Autodesk Inventor part; units mm, degrees
ref_plane "YZ Plane" through (0, 0, 0) normal (1, 0, 0) x (0, 1, 0)
ref_plane "XZ Plane" through (0, 0, 0) normal (0, 1, 0) x (-1, 0, 0)
ref_plane "XY Plane" through (0, 0, 0) normal (0, 0, 1) x (1, 0, 0)
sketch "スケッチ1" plane through (0, 0, 0) normal (1, 0, 0) x (0, 1, 0)
  circle A0 centre (0, 0) radius 10
  circle A1 centre (0, -10) radius 1.35
  circle A2 centre (8.6603, 5) radius 1.35
  circle A3 centre (-8.6603, 5) radius 1.35
  circle A4 centre (0, 0) radius 5
  line L0 (0, 0) -> (0, 50)
  circle A5 centre (0, 50) radius 22.5
  circle A6 centre (0, 0) radius 14
  line L1 (-14, 0) -> (-22.5, 50)
  line L2 (14, 0) -> (22.5, 50)
  line L3 (0, -14) -> (-11.62, -14)
  line L4 (-11.62, -14) -> (-14, 0)
  line L5 (0, -14) -> (11.62, -14)
  line L6 (11.62, -14) -> (14, 0)
  line L7 (0, 20) -> (-17.4, 20)
  line L8 (0, 20) -> (17.4, 20)
  dimension "d0" = 20
  dimension "d1" = 2.7
  dimension "d4" = 360
  dimension "d6" = 10
  dimension "d7" = 50
  dimension "d8" = 45
  dimension "d9" = 28
extrude "押し出し1" add sketch "スケッチ1" along normal blind 3 contours A0 A1 A3 A2 | A6 L6 L4 | A6 L1 L7 L0 | L0 L8 L2 A6 | L6 L5 A6 | A6 L3 L4
sketch "スケッチ2" plane through (0, -17.4, 20) normal (0, 0, 1) x (1, 0, 0)
  line L0 (0, 17.4) -> (30, 17.4)
  circle A0 centre (30, 17.4) radius 22.5
  circle A1 centre (30, 17.4) radius 18.5
  circle A2 centre (30, 17.4) radius 14
  circle A3 centre (48.5, 17.4) radius 1.35
  circle A4 centre (20.75, 33.4215) radius 1.35
  circle A5 centre (20.75, 1.3785) radius 1.35
  line L1 (0, 29.02) -> (0, 34.8)
  line L2 (0, 0) -> (0, 5.78)
  line L3 (0, 34.8) -> (0, 0)
  line L4 (3, 29.02) -> (3, 34.8)
  line L5 (3, 34.8) -> (6, 34.8)
  line L6 (6, 34.8) -> (30, 39.9)
  line L7 (3, 0) -> (3, 5.78)
  line L8 (3, 0) -> (6, 0)
  line L9 (6, 0) -> (30, -5.1)
  line L10 (3, 0) -> (0, 0)
  line L11 (0, 34.8) -> (3, 34.8)
  line L12 (0, 0) -> (0, 34.8)
  line L13 (0, 34.8) -> (3, 34.8)
  dimension "d14" = 37
  dimension "d12" = 30
  dimension "d13" = 45
  dimension "d15" = 28
  dimension "d16" = 2.7
  dimension "d19" = 360
  dimension "d21" = 3
  dimension "d22" = 3
extrude "押し出し2" add sketch "スケッチ2" along normal blind 3 contours L3 L1 L11 L5 L6 A0 L0 | L0 A0 L9 L8 L10 L2 L3 | A1 A4 A3 A5 | A0 L6 L9
fillet "フィレット1" radius 3 2 edges at (3, 0, 20) (0, 0, 23)
fillet "フィレット2" radius 3 2 edges at (1.5, -11.62, -14) (1.5, 11.62, -14)
sketch "スケッチ3" plane through (0, -17.4, 23) normal (0, 0, 1) x (1, 0, 0)
  arc A0 (30, -5.1) -> (30, 39.9) centre (30, 17.4) ccw
  line L0 (30, 17.4) -> (150, 17.4)
  circle A1 centre (150, 17.4) radius 10
  line L1 (150, 27.4) -> (50.1556, 27.4)
  line L2 (150, 7.4) -> (50.1556, 7.4)
  circle A2 centre (150, 17.4) radius 3
  line L3 (150, 17.4) -> (150, 16.4)
  line L4 (150, 16.4) -> (154.5, 16.4)
  line L5 (150, 17.4) -> (149, 17.4)
  line L6 (149, 17.4) -> (149, 21.9)
  arc A3 (154.5, 16.4) -> (149, 21.9) centre (149.3141, 16.7141) ccw
  point P0 (0, 17.4)
  dimension "d27" = 120
  dimension "d28" = 20
  dimension "d29" = 6
  dimension "d32" = 1
  dimension "d33" = 4.5
  dimension "d34" = 1
  dimension "d35" = 4.5
extrude "押し出し3" add sketch "スケッチ3" against normal blind 3 contours A0 L0 A1 L2 | A0 L1 A1 L0 | A1 | L6 A3 L4 A2
sketch "スケッチ4" plane through (0, -17.4, 23) normal (0, 0, 1) x (1, 0, 0)
  circle A0 centre (150, 17.4) radius 3
  line L0 (150, 17.4) -> (150, 16.4)
  line L1 (150, 16.4) -> (154.5, 16.4)
  line L2 (150, 17.4) -> (154.5, 17.4)
  line L3 (150, 17.4) -> (149, 17.4)
  line L4 (149, 17.4) -> (149, 21.9)
  line L5 (150, 17.4) -> (150, 21.9)
  line L6 (149, 21.9) -> (150, 21.9)
  line L7 (154.5, 17.4) -> (154.5, 16.4)
  arc A1 (154.5, 17.4) -> (150, 21.9) centre (150, 17.4) ccw
  point P0 (0, 17.4)
  point P1 (149, 20.2284)
  point P2 (152.8284, 16.4)
  dimension "d36" = 1
  dimension "d37" = 4.5
  dimension "d38" = 1
  dimension "d39" = 4.5
extrude "押し出し4" cut sketch "スケッチ4" against normal blind 3 contours L2 L7 L1 A0 | A0 L5 A1 L2 | A0 L4 L6 L5
sketch "スケッチ5" plane through (0, -17.4, 23) normal (0, 0, 1) x (1, 0, 0)
  circle A0 centre (132, 25.4) radius 1
  circle A1 centre (128, 25.4) radius 1
  point P0 (0, 17.4)
  dimension "d42" = 2
  dimension "d43" = 2
extrude "押し出し5" cut sketch "スケッチ5" against normal blind 3
thread "ねじ1"
thread "ねじ2"
sketch "スケッチ6" plane through (0, -17.4, 20) normal (0, 0, -1) x (-1, 0, 0)
  line L0 (-50.1556, 27.4) -> (-150, 27.4)
  line L1 (-130, 27.4) -> (-125, 27.4)
  line L2 (-125, 27.4) -> (-125, 22.4)
  line L3 (-125, 22.4) -> (-135, 22.4)
  line L4 (-135, 22.4) -> (-135, 27.4)
  line L5 (-135, 27.4) -> (-130, 27.4)
  point P0 (0, 17.4)
  dimension "d50" = 5
  dimension "d51" = 5
  dimension "d52" = 10
extrude "押し出し6" cut sketch "スケッチ6" against normal blind 1
properties part number "motor_holder_1" material "アルミニウム 6061"
Verification items for the finished model (mm, model axes). A direction names the side the tool comes from. Coordinates: 2 decimals unless noted, no trailing zeros. Order: outer loops, then holes, each group sorted by start corner. A loop starts at its lowest first (then second) coordinate and runs counter-clockwise, first axis right, second up.
1. Scan lines: line 1 (Y direction, x = 128, z = 21.65); line 2 (Z direction, x = 81, y = -6); line 3 (X direction, y = -9, z = 17). Record each from-to range of solid material in increasing order.
Results found:
line 1: y = -10 to 7, 9 to 10
line 2: z = 20 to 23
line 3: x = 0 to 3
2. Release check for a two-part mould opening along Y. For faces 1 (the face through (0.86, 0.24, 22.1)), 2 (the face through (153.217, 3.147, 21.521)), 3 (the face through (160, 0, 22)) record: +Y half, -Y half, draft (parallel to the pull), parting line (faces both ways), or undercut.
Results found:
face 1: draft
face 2: undercut
face 3: parting line
3. Set-up check for faces 4 (the face through (3, -0.2, 5.2)), 5 (the face through (63, 0, 23)), 6 (the face through (147.82, -2.06, 21.52)), 7 (the face through (101, -10, 22)), 8 (the face through (101, 10, 22)): record each of +Z, -Z, +X, -X, +Y, -Y from which the full face is reachable in a straight line by a thin tool's end or side.
Results found:
face 4: -Z, +X, +Y, -Y
face 5: +Z, +X, -X, +Y, -Y
face 6: +Z, -Z
face 7: +Z, -Z, +X, -Y
face 8: +Z, -Z, +X, +Y
4. Go/stop test with flat-tipped pins: pin 1 Ø0.8 at (x, z) = (149.5, 22) entering from -Y; pin 2 Ø3.5 at (x, z) = (1.5, 21.5) entering from +Y; pin 3 Ø6 at (x, z) = (52, 18.5) entering from -Y; pin 4 Ø1.2 at (x, y) = (128, 8) entering from -Z. Record where each tip stops, or that it passes through.
Results found:
pin 1: stops at y = -10
pin 2: stops at y = 17.4
pin 3: stops at y = -11.39
pin 4: passes through
5. Sectioned sample at A-A, the plane z = 8. Record the cut outline in (x, y), and give its area (3 significant figures).
Results found:
outline: (0, -15.36) - (3, -15.36) - (3, 15.36) - (0, 15.36) - close
area: 92.2 mm2
6. Sectioned sample at B-B, the plane x = 118.5. Record the cut outline in (y, z), and give its area (3 significant figures).
Results found:
outline: (-10, 20) - (10, 20) - (10, 23) - (-10, 23) - close
area: 60.0 mm2
